Input: part model. Units: mm. Frame: model coordinates. Face numbers are marked on the shaded views. A direction names the side the tool comes from. Give positions to 0.01 mm unless a question says otherwise; leave off trailing zeros. Write each loop counter-clockwise with the first axis right and the second up, starting at its lowest first coordinate (ties: lowest second). Pieces come first, ordered by that corner, then holes.
```python
from build123d import *

# Parameters (mm, degrees)
SKETCH1_R           = 18.5
SKETCH1_R_2         = 8.5
BOSS_EXTRUDE1_DEPTH = 8
SKETCH2_W           = 16
SKETCH2_H           = 83.319172682
BOSS_EXTRUDE2_DEPTH = 8
SKETCH3_W           = 16
SKETCH3_H           = 83.319172682
BOSS_EXTRUDE3_DEPTH = 8
SKETCH4_W           = 4
SKETCH4_H           = 2.038644179
CUT_EXTRUDE3_DEPTH  = 103.947802308
FILLET1_R           = 10
SKETCH5_R           = 3
CUT_EXTRUDE4_DEPTH  = 104.760541633


with BuildPart() as part:
    # Sketch1 → Boss-Extrude1 (new, symmetric)
    with BuildSketch(Plane.XY):
        Circle(SKETCH1_R)
        Circle(SKETCH1_R_2, mode=Mode.SUBTRACT)
    extrude(amount=BOSS_EXTRUDE1_DEPTH, both=True)

    # Sketch2 → Boss-Extrude2 (add, symmetric)
    with BuildSketch(Plane.XY):
        with Locations((0, 58.340413659)):
            Rectangle(SKETCH2_W, SKETCH2_H)
    extrude(amount=BOSS_EXTRUDE2_DEPTH, both=True)

    # Sketch3 → Boss-Extrude3 (add, symmetric)
    with BuildSketch(Plane.XY):
        with Locations((0, -58.340413659)):
            Rectangle(SKETCH3_W, SKETCH3_H)
    extrude(amount=BOSS_EXTRUDE3_DEPTH, both=True)

    # Sketch4 → Cut-Extrude3 (cut, through all)
    with BuildSketch(Plane(origin=(0, 0, -8), x_dir=(-1, 0, 0), z_dir=(0, 0, -1))):
        with Locations((0, 9.28067791)):
            Rectangle(SKETCH4_W, SKETCH4_H)
    extrude(amount=-CUT_EXTRUDE3_DEPTH, mode=Mode.SUBTRACT)

    # Fillet1
    fillet1_edges = [part.edges().sort_by_distance(p)[0] for p in [
        (8, 16.680827318, 0),
        (-8, 16.680827318, 0),
        (8, -16.680827318, 0),
        (-8, -16.680827318, 0),
    ]]
    fillet(fillet1_edges, radius=FILLET1_R)

    # Sketch5 → Cut-Extrude4 (cut, through all)
    with BuildSketch(Plane(origin=(8, 0, 0), x_dir=(0, 0, -1), z_dir=(1, 0, 0))):
        with Locations(Location((0, 90, 0), (0, 0, 90))):
            Circle(SKETCH5_R)
        with Locations(Location((0, 70, 0), (0, 0, 90))):
            Circle(SKETCH5_R)
        with Locations(Location((0, -70, 0), (0, 0, 90))):
            Circle(SKETCH5_R)
        with Locations(Location((0, -90, 0), (0, 0, 90))):
            Circle(SKETCH5_R)
    extrude(amount=-CUT_EXTRUDE4_DEPTH, mode=Mode.SUBTRACT)


solid = part.part
```
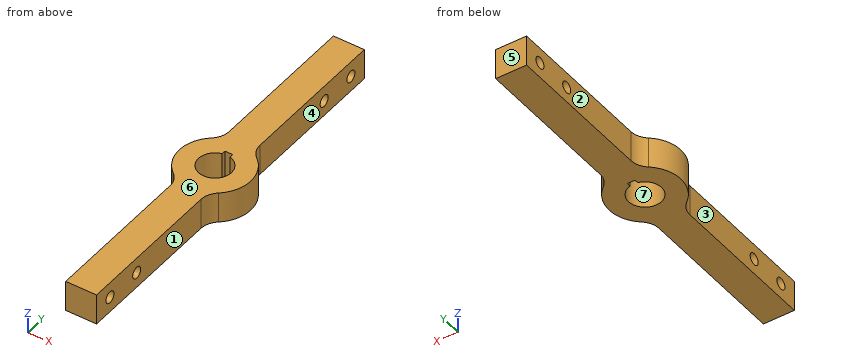
Q1. Section C-C, the plane z = 5.5. Return the cut outline in (x, y).
Q2. Access query for the marked faces 1, 2, 3 and 4. Directions: +Z, -Z, +X, -X, +Y, -Y. A direction counts if a zero-diameter tool reaches every point of the face in a straight line with its end or side. Return the directions, or none.
Q3. Section B-B, the plane y = -90. Return the cut outline in (x, z).
Q4. Mould query, pull axis Y, two halves, no side actions, for the marked faces 5, 6 and 7. Classes: +Y half, -Y half, draft (parallel to the pull), parting line (faces both ways), or undercut.
Q5. Section A-A, the plane x = 0. Return the cut outline in (y, z), then the cut area to 3 significant figures.
Q6. Section D-D, the plane y = -69.5. Return the cut outline in (x, z), then the cut area to 3 significant figures.
Q7. Material intervals for line 1 along Z through (x, y) = (0.5, 70); line 2 along Y through (x, z) = (0.5, -1); line 3 along Y through (x, z) = (-6, -1), sorted ascending.
Q8. Pin query (flat end, axial travel): pin 1 (9.5 mm diameter, centred on y = 90, z = 0, fed in from +X); pin 2 (0.6 mm diameter, centred on y = 9, z = 0.5, fed in from +X); pin 3 (2 mm diameter, centred on y = 10, z = 3, fed in from -X); pin 4 (6 mm diameter, centred on x = -0.5, y = 3, fed in from -Z). Return the tip coordinate at first contact, or that it passes through.
Solutions:
1. outline: (-11.68, -14.34) arc R10 cw to (-8, -22.1) - (-8, -100) - (8, -100) - (8, -22.1) arc R10 cw to (11.68, -14.34) arc R18.5 ccw to (11.68, 14.34) arc R10 cw to (8, 22.1) - (8, 100) - (-8, 100) - (-8, 22.1) arc R10 cw to (-11.68, 14.34) arc R18.5 ccw to start; hole (-2, 8.26) arc R8.5 ccw (long way) to (2, 8.26) - (2, 10.3) - (-2, 10.3) - close
2. face 1: +Z, -Z, +X, -Y
2. face 2: +Z, -Z, -X, +Y
2. face 3: +Z, -Z, -X, -Y
2. face 4: +Z, -Z, +X, +Y
3. outline: (-8, -8) - (8, -8) - (8, -3) - (-8, -3) - close; (-8, 3) - (8, 3) - (8, 8) - (-8, 8) - close
4. face 5: +Y half
4. face 6: draft
4. face 7: undercut
5. outline: (-100, -8) - (-8.5, -8) - (-8.5, 8) - (-100, 8) - close; (10.3, -8) - (100, -8) - (100, 8) - (10.3, 8) - close; hole circle Ø6 at (-90, 0); hole circle Ø6 at (-70, 0); hole circle Ø6 at (70, 0); hole circle Ø6 at (90, 0)
5. area: 2,790 mm2
6. outline: (-8, -8) - (8, -8) - (8, -2.96) - (-8, -2.96) - close; (-8, 2.96) - (8, 2.96) - (8, 8) - (-8, 8) - close
6. area: 161 mm2
7. line 1: z = -8 to -3, 3 to 8
7. line 2: y = -100 to -92.83, -87.17 to -72.83, -67.17 to -8.49, 10.3 to 67.17, 72.83 to 87.17, 92.83 to 100
7. line 3: y = -100 to -92.83, -87.17 to -72.83, -67.17 to -6.02, 6.02 to 67.17, 72.83 to 87.17, 92.83 to 100
8. pin 1: stops at x = 8
8. pin 2: stops at x = 16.33
8. pin 3: stops at x = -16.16
8. pin 4: passes through
